Job drawing, mm, ordinate dimensions from the low corner. One solid piece. A direction names the side the tool comes from. Coordinates: 2 decimals unless noted, no trailing zeros. Order: outer loops, then holes, each group sorted by start corner. A loop starts at its lowest first (then second) coordinate and runs counter-clockwise, first axis right, second up. Notation, with made-up numbers: (-8.75, 28.25) - (27.25, 28.25) arc R24 ccw to (27.25, 43.25) - close; hole circle Ø1 at (76, 38). An arc over 180 degrees is marked (long way). Return JSON: item names as keys, results as strings.
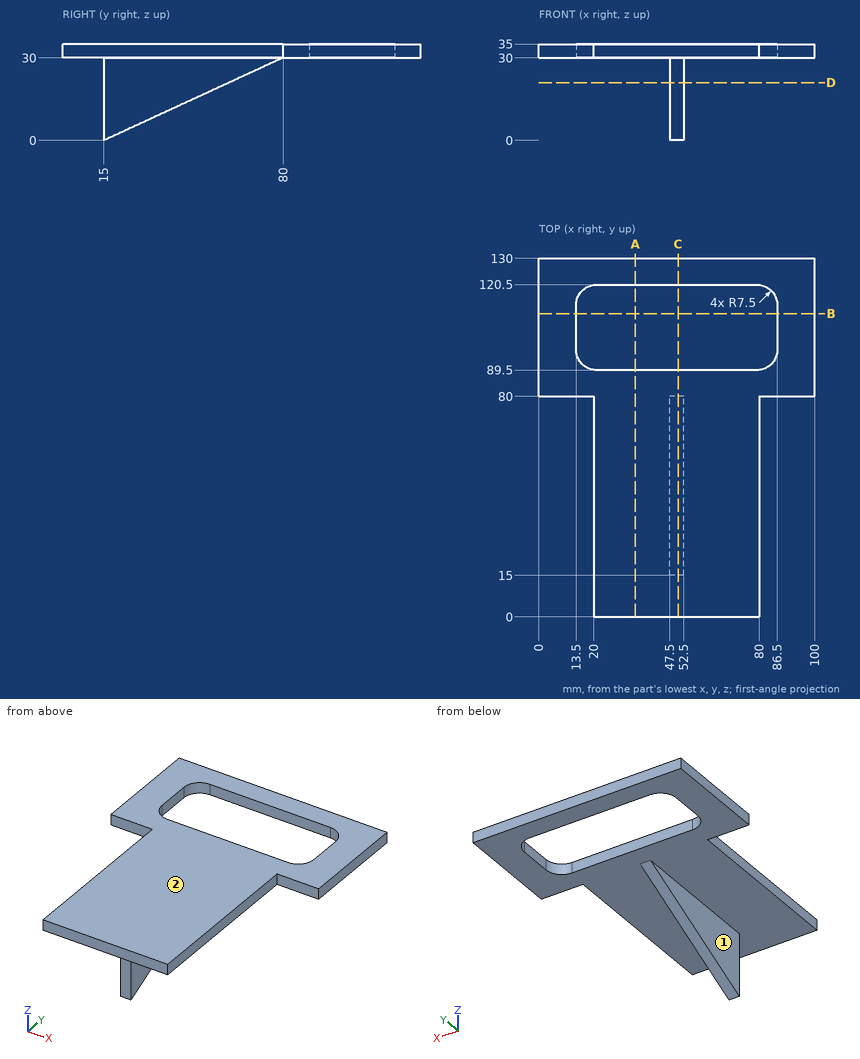
1. Cut at C-C on x = 50.5. Give the cut face in (y, z), plus the area to 3 significant figures.
Check values:
{"outline": "(0, 30) - (15, 30) - (15, 0) - (80, 30) - (89.5, 30) - (89.5, 35) - (0, 35) - close; (120.5, 30) - (130, 30) - (130, 35) - (120.5, 35) - close", "area": "1,470 mm²"}
2. Drop flat-ended pins along their axis: pin 1 (15 mm diameter, centred on y = 49, z = 12.5, fed in from +X); pin 2 (2 mm diameter, centred on x = 79, y = 40, fed in from -Z); pin 3 (2.5 mm diameter, centred on x = 6.5, z = 33.5, fed in from -Y). Give the stop position or say it passes through.
Check values:
{"pin 1": "x = 52.5", "pin 2": "z = 30", "pin 3": "y = 80"}
3. Cut at D-D on z = 21. Give the cut face in (x, y).
Check values:
{"outline": "(47.5, 15) - (52.5, 15) - (52.5, 60.5) - (47.5, 60.5) - close"}
4. Cut at B-B on y = 110. Give the cut face in (x, z).
Check values:
{"outline": "(0, 30) - (13.5, 30) - (13.5, 35) - (0, 35) - close; (86.5, 30) - (100, 30) - (100, 35) - (86.5, 35) - close"}
5. Cut at A-A on x = 35. Give the cut face in (y, z).
Check values:
{"outline": "(0, 30) - (89.5, 30) - (89.5, 35) - (0, 35) - close; (120.5, 30) - (130, 30) - (130, 35) - (120.5, 35) - close"}
6. Tool access for the marked faces 1 and 2: list every direction of +Z, -Z, +X, -X, +Y, -Y with a clear straight run to the whole face (end or side of a thin tool).
Check values:
{"face 1": "-Z, -X, +Y, -Y", "face 2": "+Z, +X, -X, +Y, -Y"}
7. Probe L1, parallel to Y at x = 56, z = 32; L2, parallel to Z at x = 60.5, y = 75.5; L3, parallel to Y at x = 12.5, z = 34.5. List the from-to ranges inside material, lowest first.
Check values:
{"L1": "0 to 89.5, 120.5 to 130", "L2": "30 to 35", "L3": "80 to 130"}
